Design review of the part built by this model. Coordinates are the model's own, in mm. Coordinates: 2 decimals unless noted, no trailing zeros. Loops run counter-clockwise (first coordinate to the right, second up) from the corner with the lowest first, then second, coordinate; pieces in that order, holes last. Notation, with made-up numbers: M 63,15 L 88,15 A22 cw 88,24 Z; hole C 78.25,47 d1. An arc over 180 degrees is marked long. One line per item, written item: value.
```python
from build123d import *

# Parameters (mm, degrees)
F0_R     = 25.4
F0_R_2   = 22.86
F1_DEPTH = 2.54
F2_R     = 0.635
F3_R     = 0.635
F4_R     = 0.635


with BuildPart() as f1:
    # F0 (on Front) → F1 (new body)
    with BuildSketch(Plane.XZ):
        Circle(F0_R)
        Circle(F0_R_2, mode=Mode.SUBTRACT)
    extrude(amount=F1_DEPTH)

    # F2
    f2_edges = [f1.edges().sort_by_distance(p)[0] for p in [
        (-22.86, -2.54, 0),
    ]]
    fillet(f2_edges, radius=F2_R)

    # F3
    f3_edges = [f1.edges().sort_by_distance(p)[0] for p in [
        (-25.4, -2.54, 0),
    ]]
    fillet(f3_edges, radius=F3_R)

    # F4
    f4_edges = [f1.edges().sort_by_distance(p)[0] for p in [
        (-25.4, 0, 0),
        (-22.86, 0, 0),
    ]]
    fillet(f4_edges, radius=F4_R)


solid = f1.part
```
(1) We need section A-A on z = 0. State the section outline as (x, y) points (3 decimals).
Reply:
outline: M -25.4,-1.905 A0.635 ccw -24.765,-2.54 L -23.495,-2.54 A0.635 ccw -22.86,-1.905 L -22.86,-0.635 A0.635 ccw -23.495,0 L -24.765,0 A0.635 ccw -25.4,-0.635 Z; M 22.86,-1.905 A0.635 ccw 23.495,-2.54 L 24.765,-2.54 A0.635 ccw 25.4,-1.905 L 25.4,-0.635 A0.635 ccw 24.765,0 L 23.495,0 A0.635 ccw 22.86,-0.635 Z
(2) Mouldability with a two-part tool opening along Z and no side actions: class faces 1 (the cylindrical face through (-5.506, -1.261, -24.796)), 2 (the cylindrical face through (21.804, -1.261, 6.867)), 3 (the flat face through (9, 0, -22)) as released by +Z, released by -Z, zero draft, split by the parting line, or undercut.
Reply:
face 1: split by the parting line
face 2: undercut
face 3: zero draft
(3) To check wall thickness, follow line 1 along Z through (x, y) = (0, -0.9); line 2 along Z through (x, y) = (-16.5, -1.35); line 3 along X through (y, z) = (-2.4, 12). State the ranges of each line that lie inside material, in increasing order. Write a range as [from, to].
Reply:
line 1: z = [-25.4, -22.86], [22.86, 25.4]
line 2: z = [-19.31, -15.82], [15.82, 19.31]
line 3: x = [-22.12, -19.74], [19.74, 22.12]
(4) We need section B-B on x = 0. State the section outline as (y, z) points (3 decimals).
Reply:
outline: M -2.54,-24.765 A0.635 ccw -1.905,-25.4 L -0.635,-25.4 A0.635 ccw 0,-24.765 L 0,-23.495 A0.635 ccw -0.635,-22.86 L -1.905,-22.86 A0.635 ccw -2.54,-23.495 Z; M -2.54,23.495 A0.635 ccw -1.905,22.86 L -0.635,22.86 A0.635 ccw 0,23.495 L 0,24.765 A0.635 ccw -0.635,25.4 L -1.905,25.4 A0.635 ccw -2.54,24.765 Z
(5) Insertion check: pin 1 (1 mm diameter, centred on y = -0.5, z = 19.5, fed in from -X). The pin has a flat end and moves straight along its axis. Give the tip position at first contact, or say it passes through.
Reply:
pin 1: stops at x = -16.85
